For this review, take the finished solid that the model builds, in its own axes (mm). A direction names the side the tool comes from. Give positions to 0.01 mm unless a question says otherwise; leave off trailing zeros. Order: outer loops, then holes, each group sorted by start corner. A loop starts at its lowest first (then second) coordinate and runs counter-clockwise, first axis right, second up.
Item 1: Consider section B-B (x = 43.5). Give the boundary of the cut face in (y, z) (3 decimals), plus the area to 3 significant figures.
Item 2: Machinability: for faces 5 (the flat face through (35.224, 10, -29)), 6 (the flat face through (43.97, 0.74, -23.35)), 7 (the flat face through (15.984, 10, -29)), 8 (the flat face through (33.224, 10, -28)), 9 (the flat face through (51.131, 10, -16)), which of the approach directions +Z, -Z, +X, -X, +Y, -Y give a long, thin tool a straight path to every point of the face, cutting with its end or side? Answer none if there is none.
Item 3: The part is to be moulded in two halves that separate along Z. For faces 1 (the flat face through (34, 10, 0)), 2 (the flat face through (42, 10, -22.534)), 3 (the flat face through (25, 2, -17)), 4 (the flat face through (52.12, 9.8, -23.12)), say which applies: released by +Z, released by -Z, zero draft, split by the parting line, or undercut.
Item 4: Consider section C-C (x = 36). Give the boundary of the cut face in (y, z) (3 decimals).
Item 5: For probe 1 along Z at (x, y) = (40, 17); probe 2 along X at (y, z) = (11.5, -15); probe 3 along X at (y, z) = (12.5, -9), list the stretches that pass through material, from the lowest coordinate up.
Item 6: For P1, Ø1.1, axis at y = 8, z = -2.5, coming from the +X side; P2, Ø7, axis at x = 46.5, y = 8, coming from the -Z side; P3, Ø6, axis at y = 13, z = -29, coming from the -X side, all flat-tipped, find the tip position at first contact; note any pin that passes through.
Item 7: Consider section A-A (z = -16). Give the boundary of the cut face in (x, y) (1 decimal).
```python
from build123d import *

# Parameters (mm, degrees)
SKETCH1_R           = 2.159
BOSS_EXTRUDE1_DEPTH = 2
BOSS_EXTRUDE2_DEPTH = 15.875
CHAMFER1_SIZE       = 2
CHAMFER2_SIZE       = 2
CHAMFER3_SIZE       = 1.5
CHAMFER4_SIZE       = 1.5
CHAMFER5_SIZE       = 1.5


with BuildPart() as part:
    # Sketch1 → Boss-Extrude1 (new body)
    with BuildSketch(Plane(origin=(0, 0, 0), x_dir=(1, 0, 0), z_dir=(0, 1, 0))):
        Polygon((35.223504259, 33.533672595), (15.983504259, 33.533672595), (15.983504259, 24.107172595), (-1.923495741, 24.107172595), (-1.923495741, 5.411272595), (15.983504259, 5.411272595), (15.983504259, -0.278017555), (35.223504259, -0.278017555), (35.223504259, 5.411272595), (53.130504259, 5.411272595), (53.130504259, 24.107172595), (35.223504259, 24.107172595), align=None)
        with Locations(Location((16.078504259, 16.056672595, 0), (0, 0, 270))):
            Circle(SKETCH1_R, mode=Mode.SUBTRACT)
        with Locations(Location((35.128504259, 16.056672595, 0), (0, 0, 270))):
            Circle(SKETCH1_R, mode=Mode.SUBTRACT)
    extrude(amount=BOSS_EXTRUDE1_DEPTH)

    # Sketch3 → Boss-Extrude2 (add)
    with BuildSketch(Plane(origin=(0, 2, 0), x_dir=(1, 0, 0), z_dir=(0, 1, 0))):
        Polygon((33.223504259, 30.817862745), (33.223504259, 33.533672595), (35.223504259, 33.533672595), (35.223504259, 24.107172595), (53.130504259, 24.107172595), (53.130504259, 5.411272595), (35.223504259, 5.411272595), (35.223504259, -0.278017555), (33.223504259, -0.278017555), (33.223504259, 1.721982445), (33.223504259, 9.579672595), (51.130504259, 9.579672595), (51.130504259, 22.533672595), (33.223504259, 22.533672595), align=None)
        Polygon((17.983504259, 1.721982445), (17.983504259, -0.278017555), (15.983504259, -0.278017555), (15.983504259, 5.411272595), (-1.923495741, 5.411272595), (-1.923495741, 24.107172595), (15.983504259, 24.107172595), (15.983504259, 33.533672595), (17.983504259, 33.533672595), (17.983504259, 29.040712972), (17.983504259, 22.533672595), (0.076504259, 22.533672595), (0.076504259, 9.579672595), (17.983504259, 9.579672595), align=None)
    extrude(amount=BOSS_EXTRUDE2_DEPTH)

    # Chamfer1
    chamfer1_edges = [part.edges().sort_by_distance(p)[0] for p in [
        (53.130504259, 8.9375, -24.107172595),
        (53.130504259, 8.9375, -5.411272595),
        (-1.923495741, 8.9375, -5.411272595),
        (-1.923495741, 8.9375, -24.107172595),
    ]]
    chamfer(chamfer1_edges, length=CHAMFER1_SIZE)

    # Chamfer2
    chamfer2_edges = [part.edges().sort_by_distance(p)[0] for p in [
        (35.223504259, 8.9375, -24.107172595),
        (35.223504259, 8.9375, -5.411272595),
        (15.983504259, 8.9375, -5.411272595),
        (15.983504259, 8.9375, -24.107172595),
    ]]
    chamfer(chamfer2_edges, length=CHAMFER2_SIZE)

    # Chamfer3
    chamfer3_edges = [part.edges().sort_by_distance(p)[0] for p in [
        (15.983504259, 8.9375, -33.533672595),
        (35.223504259, 8.9375, -33.533672595),
    ]]
    chamfer(chamfer3_edges, length=CHAMFER3_SIZE)

    # Chamfer4
    chamfer4_edges = [part.edges().sort_by_distance(p)[0] for p in [
        (35.223504259, 8.9375, 0.278017555),
        (15.983504259, 8.9375, 0.278017555),
    ]]
    chamfer(chamfer4_edges, length=CHAMFER4_SIZE)

    # Chamfer5
    chamfer5_edges = [part.edges().sort_by_distance(p)[0] for p in [
        (53.130504259, 0, -14.759222595),
        (44.177004259, 0, -24.107172595),
        (7.030004259, 0, -5.411272595),
        (-1.923495741, 0, -14.759222595),
        (-0.923495741, 0, -6.411272595),
        (-0.923495741, 0, -23.107172595),
        (52.130504259, 0, -23.107172595),
        (52.130504259, 0, -6.411272595),
        (44.177004259, 0, -5.411272595),
        (15.983504259, 0, -2.31662752),
        (7.030004259, 0, -24.107172595),
        (35.223504259, 0, -29.070422595),
        (36.223504259, 0, -4.411272595),
        (14.983504259, 0, -4.411272595),
        (14.983504259, 0, -25.107172595),
        (36.223504259, 0, -25.107172595),
        (15.983504259, 0, -29.070422595),
        (25.603504259, 0, -33.533672595),
        (34.473504259, 0, -32.783672595),
        (16.733504259, 0, -32.783672595),
        (25.603504259, 0, 0.278017555),
        (35.223504259, 0, -2.31662752),
        (34.473504259, 0, -0.471982445),
        (16.733504259, 0, -0.471982445),
    ]]
    chamfer(chamfer5_edges, length=CHAMFER5_SIZE)


solid = part.part
```
Resolved:
1. outline: (0, -22.607) - (1.5, -24.107) - (17.875, -24.107) - (17.875, -22.534) - (2, -22.534) - (2, -9.58) - (17.875, -9.58) - (17.875, -5.411) - (1.5, -5.411) - (0, -6.911) - close
1. area: 126 mm2
2. face 5: -Z, +X, +Y, -Y
2. face 6: -Z, +X, -Y
2. face 7: -Z, -X, +Y, -Y
2. face 8: +Z, -Z, +Y
2. face 9: +Y
3. face 1: released by +Z
3. face 2: undercut
3. face 3: undercut
3. face 4: released by -Z
4. outline: (0, -23.209) - (1.5, -25.331) - (17.875, -25.331) - (17.875, -22.534) - (2, -22.534) - (2, -18.032) - (0, -18.032) - close; (0, -14.081) - (2, -14.081) - (2, -9.58) - (17.875, -9.58) - (17.875, -4.188) - (1.5, -4.188) - (0, -6.309) - close
5. probe 1: z = -24.11 to -22.53, -9.58 to -5.41
5. probe 2: x = -1.92 to 0.08, 51.13 to 53.13
5. probe 3: x = -1.92 to 17.98, 33.22 to 53.13
6. P1: stops at x = 35.22
6. P2: stops at z = -24.11
6. P3: stops at x = 15.88
7. outline: (-1.9, 1.5) - (-0.4, 0) - (13.9, 0) - (13.9, 2) - (0.1, 2) - (0.1, 17.9) - (-1.9, 17.9) - close; (18.2, 0) - (33, 0) - (33, 2) - (18.2, 2) - close; (37.3, 0) - (51.6, 0) - (53.1, 1.5) - (53.1, 17.9) - (51.1, 17.9) - (51.1, 2) - (37.3, 2) - close
